Can you work these out from the drawing? Everything is in mm from the part's minimum corner. A direction names the side the tool comes from. Round coordinates to 2 decimals unless told otherwise and drop trailing zeros. Order: outer loops, then holes, each group sorted by start corner. A loop starts at its lowest first (then second) coordinate and runs counter-clockwise, first axis right, second up. Notation, with made-up numbers: (50.25, -36.75) -> (94.25, -36.75) arc R5 ccw to (94.25, -28.75) -> close; hole circle Ø8 at (28.5, 22). An arc over 180 degrees is marked (long way). One line per item, written item: value.
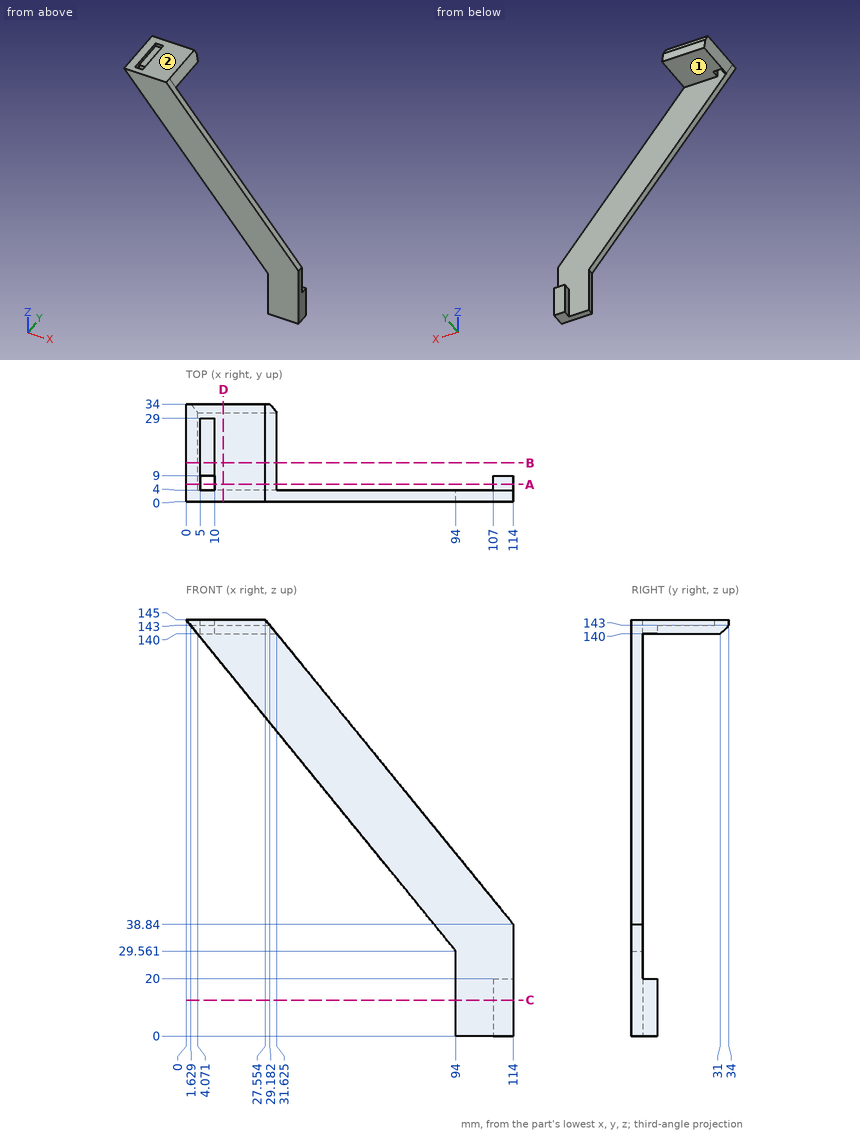
Q1. I want a section at B-B on y = 13.5. List the corners of the cut face in (x, z) for me (1 decimal).
Answers below:
outline: (0, 145) -> (4.1, 140) -> (31.6, 140) -> (27.6, 145) -> (10, 145) -> (10, 143) -> (5, 143) -> (5, 145) -> close
Q2. I want a section at C-C on z = 12.5. List the corners of the cut face in (x, y) for me.
Answers below:
outline: (94, 0) -> (114, 0) -> (114, 9) -> (107, 9) -> (107, 4) -> (94, 4) -> close
Q3. I want a section at D-D on x = 13. List the corners of the cut face in (y, z) for me (1 decimal).
Answers below:
outline: (0, 129) -> (4, 129) -> (4, 140) -> (31, 140) -> (34, 143) -> (34, 145) -> (0, 145) -> close
Q4. I want a section at A-A on y = 6. List the corners of the cut face in (x, z) for me (1 decimal).
Answers below:
outline: (0, 145) -> (4.1, 140) -> (5, 140) -> (5, 145) -> close; (10, 140) -> (31.6, 140) -> (27.6, 145) -> (10, 145) -> close; (107, 0) -> (114, 0) -> (114, 20) -> (107, 20) -> close
Q5. On a 3-axis mill with a long thin cutter (end or side, diameter ignored), from which of +Z, -Z, +X, -X, +Y, -Y can I reach the whole of each face in a straight line? I mean the marked faces 1 and 2. Say none if no direction works.
Answers below:
face 1: -Z, +X, -X, +Y
face 2: +Z, +X, -X, +Y, -Y
Q6. Please list where these lines run through material, in increasing order: line 1 along Y through (x, z) = (23, 117); line 2 along X through (y, z) = (4.5, 18.5); line 3 along Z through (x, y) = (30, 30) (1 decimal).
Answers below:
line 1: 0 to 4
line 2: 107 to 114
line 3: 140 to 142
Q7. Will these pins go through, and if not, where does the flat tip stop? pin 1 Ø1.2 at (y, z) = (3, 18.5) entering from -X; pin 2 Ø13.5 at (x, y) = (23.5, 11.5) entering from -Z; pin 3 Ø7.5 at (x, z) = (111.5, 11) entering from +Y; pin 4 Ø12 at (x, z) = (64.5, 110.5) entering from -Y.
Answers below:
pin 1: x = 94
pin 2: z = 140
pin 3: y = 9
pin 4: through
